Here's how the part is built. I have some questions about the finished solid (model axes, mm). Face numbers are marked on the shaded views. A direction names the side the tool comes from. Round coordinates to 2 decimals unless told otherwise and drop trailing zeros. Order: outer loops, then holes, each group sorted by start corner. A loop starts at its lowest first (then second) coordinate and runs counter-clockwise, first axis right, second up. Notation, with made-up numbers: M 71,51 L 98,51 A21 cw 98,77 Z; hole C 13,-14 d1. An arc over 180 degrees is marked long. Answer as CSV lines item,"result". Start each with the question number.
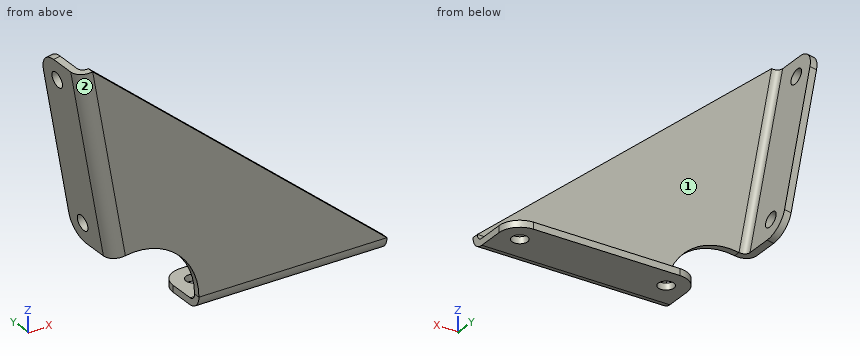
```python
from build123d import *

# Parameters (mm, degrees)
F1_DEPTH    = 2.032
F2_W        = 57.15
F2_H        = 2.032
F3_ANGLE    = 90
F4_W        = 2.032
F4_H        = 57.15
F5_ANGLE    = 90
F6_DEPTH    = 14.2875
F7_R        = 6.35
F10_D       = 4.7625
F10_ON_F8_D = 4.7625


with BuildPart() as f1:
    # F0 (on Front) → F1 (new body)
    with BuildSketch(Plane.XZ):
        with BuildLine():
            Line((-13.2319911382, 75.0423507795), (-3.3079977846, 18.7605876949))
            ThreePointArc((-3.3079977846, 18.7605876949), (12.2451039645, 14.5931466414), (19.05, 0))
            Line((19.05, 0), (76.2, 0))
            Line((76.2, 0), (-13.2319911382, 75.0423507795))
        make_face()
    extrude(amount=F1_DEPTH)

    # F2 (on face) → F3 (revolve)
    with BuildSketch(Plane(origin=(0, 0, 0), x_dir=(1, 0, 0), z_dir=(0, 0, -1))):
        with Locations((47.625, 1.016)):
            Rectangle(F2_W, F2_H)
    revolve(axis=Axis((40.305102244, 2.032, 0), (1, 0, 0)), revolution_arc=F3_ANGLE)

    # F4 (on face) → F5 (revolve)
    with BuildSketch(Plane(origin=(0, 0, 0), x_dir=(0, -1, 0), z_dir=(-0.984807753, 0, -0.1736481777))):
        with Locations((1.016, 47.625)):
            Rectangle(F4_W, F4_H)
    revolve(axis=Axis((-5.7906206967, 2.032, 32.8402418815), (0.1736481777, 0, -0.984807753)), revolution_arc=F5_ANGLE)

    # F6 (add): faces of the model
    f6_faces = [f1.faces().sort_by_distance(p)[0] for p in [
        (47.625, 2.032, -3.048),
        (-11.2716884926, 2.032, 46.3721895917),
    ]]
    extrude(f6_faces, amount=F6_DEPTH)

    # F7
    f7_edges = [f1.edges().sort_by_distance(p)[0] for p in [
        (-16.233685, 16.3195, 74.513071),
        (-6.309692, 16.3195, 18.231308),
        (19.05, 16.3195, -3.048),
        (76.2, 16.3195, -3.048),
    ]]
    fillet(f7_edges, radius=F7_R)

    # F10 (through all)
    with Locations(Plane.XY.offset(-2.032)):
        with Locations((25.4, 9.9695), (69.85, 9.9695)):
            Hole(F10_D / 2)

    # F10 on F8 (through all)
    with Locations(Plane(origin=(-2.0011293541, 0, -0.352853097), x_dir=(0, 1, 0), z_dir=(0.984807753, 0, 0.1736481777))):
        with Locations((9.9695, 25.4), (9.9695, 69.85)):
            Hole(F10_ON_F8_D / 2)


solid = f1.part
```
Item 1: If we section it at C-C on z = 15: Please give me the cut outline in (x, y), and give its area (3 significant figures).
Item 2: If I drill on line 1 along Y through (x, z) = (45.5, 8); line 2 along Z through (x, y) = (57.5, 7.5); line 3 along Y through (x, z) = (69, -3), over which ranges is the centre line in solid material (lowest first)?
Item 3: For P1, Ø6, axis at x = 15, y = 2, coming from the +Z side; P2, Ø1, axis at y = 0.5, z = 66.5, coming from the -X side; P3, Ø4.5, axis at y = 5.5, z = -2.5, coming from the -X side, each with a flat end and sliding along its axis, tell me the tip position at first contact or that it passes through.
Item 4: Which directions (+Z, -Z, +X, -X, +Y, -Y) give clear straight access to the entire face, cutting with the end or side of a thin tool? Please do the marked faces 1 and 2.
Item 5: If we section it at B-B on x = 47: Please give me the cut outline in (y, z).
Item 6: If we section it at A-A on y = 14.5: Please give me the cut outline in (x, z), and give its area (3 significant figures).
Item 7: If we section it at D-D on x = 58.5: Please give me the cut outline in (y, z), and give its area (3 significant figures).
Geometry says:
1,outline,"M 11.74,-2.03 L 58.32,-2.03 L 58.32,0 L 11.74,0 Z"
1,area,"94.7 mm²"
2,line 1,"-2.03 to 0"
2,line 2,"-4.06 to -2.03"
2,line 3,"-0.71 to 7.75, 12.19 to 16.32"
3,P1,"z = 53.23"
3,P2,"x = -15.74"
3,P3,"x = 19.05"
4,face 1,"+Z, +X, +Y"
4,face 2,"-Z, -X, -Y"
5,outline,"M -2.03,0 A4.06 ccw 2.03,-4.06 L 16.32,-4.06 L 16.32,-2.03 L 2.03,-2.03 A2.03 cw 0,0 L 0,24.5 L -2.03,24.5 Z"
6,outline,"M -16.9,72.46 L -7.64,19.93 L -5.64,20.28 L -14.9,72.82 Z; M 20.95,-4.06 L 74.3,-4.06 L 74.3,-2.03 L 20.95,-2.03 Z"
6,area,"217 mm²"
7,outline,"M -2.03,0 A4.06 ccw 2.03,-4.06 L 16.32,-4.06 L 16.32,-2.03 L 2.03,-2.03 A2.03 cw 0,0 L 0,14.85 L -2.03,14.85 Z"
7,area,"68.9 mm²"
